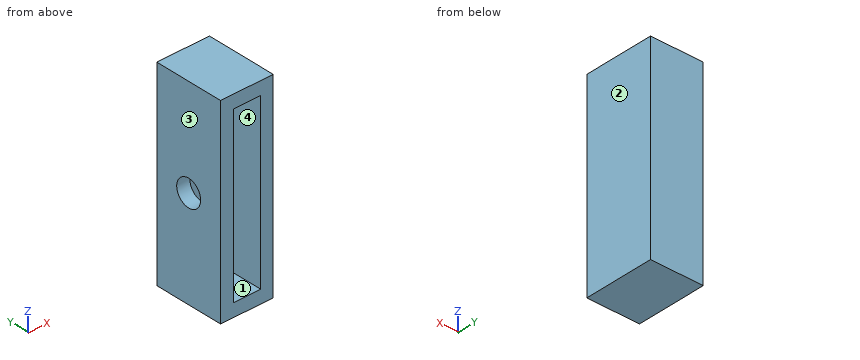
from build123d import *

# Parameters (mm, degrees)
F0_W     = 304.8
F0_H     = 1143
F1_DEPTH = 406.4
F2_W     = 156.097188
F2_H     = 990.6
F3_DEPTH = 381
F4_R     = 76.2
F5_DEPTH = 76.2


with BuildPart() as f1:
    # F0 (on Front) → F1 (new body)
    with BuildSketch(Plane.XZ):
        Rectangle(F0_W, F0_H)
    extrude(amount=F1_DEPTH)

    # F2 (on face) → F3 (cut)
    with BuildSketch(Plane.XZ.offset(406.4)):
        with Locations((1.848594, 0)):
            Rectangle(F2_W, F2_H)
    extrude(amount=-F3_DEPTH, mode=Mode.SUBTRACT)

    # F4 (on face) → F5 (cut)
    with BuildSketch(Plane(origin=(-152.4, 0, 0), x_dir=(0, -1, 0), z_dir=(-1, 0, 0))):
        with Locations((203.2, 0)):
            Circle(F4_R)
    extrude(amount=-F5_DEPTH, mode=Mode.SUBTRACT)


solid = f1.part
CAD build for the part. Positions are in the model's coordinates, mm. Face numbers are marked on the shaded views. Round coordinates to 2 decimals unless told otherwise and drop trailing zeros. Order: outer loops, then holes, each group sorted by start corner. A loop starts at its lowest first (then second) coordinate and runs counter-clockwise, first axis right, second up. Notation, with made-up numbers: (7.25, 15) -> (15.25, 15) arc R37 ccw to (15.25, 51) -> close; hole circle Ø3 at (40, -12). An arc over 180 degrees is marked (long way). Write item = value, one per line. Start each with the question number.
(1) Pull direction X, two halves, no side cores. Call the marked faces 1, 2, 3 and 4: released by +X, released by -X, zero draft, split by the parting line, or undercut.
(2) Probe line 1 (X direction, y = -309, z = -451); line 2 (Z direction, x = -56, y = -90); line 3 (Z direction, x = -123, y = -203.2). List the from-to ranges inside material, lowest first. Write a range as [from, to].
(3) Cut at A-A, the plane z = 0. List the corners of the cut face in (x, y), then the cut area to 3 significant figures.
(4) Cut at C-C, the plane x = 5.5. List the corners of the cut face in (y, z), then the cut area to 3 significant figures.
(5) Cut at D-D, the plane y = -203.2. List the corners of the cut face in (x, z).
(6) Cut at B-B, the plane y = -105. List the corners of the cut face in (x, z), then the cut area to 3 significant figures.
Model answer:
q1.face_1 = undercut
q1.face_2 = released by +X
q1.face_3 = released by -X
q1.face_4 = undercut
q2.line_1 = [-152.4, -76.2], [79.9, 152.4]
q2.line_2 = [-571.5, -495.3], [495.3, 571.5]
q2.line_3 = [-571.5, -76.2], [76.2, 571.5]
q3.outline = (-152.4, -406.4) -> (-76.2, -406.4) -> (-76.2, -279.4) -> (-152.4, -279.4) -> close; (-152.4, -127) -> (-76.2, -127) -> (-76.2, -25.4) -> (79.9, -25.4) -> (79.9, -406.4) -> (152.4, -406.4) -> (152.4, 0) -> (-152.4, 0) -> close
q3.area = 52,800 mm2
q4.outline = (-406.4, -571.5) -> (0, -571.5) -> (0, 571.5) -> (-406.4, 571.5) -> (-406.4, 495.3) -> (-25.4, 495.3) -> (-25.4, -495.3) -> (-406.4, -495.3) -> close
q4.area = 87,100 mm2
q5.outline = (-152.4, -571.5) -> (152.4, -571.5) -> (152.4, 571.5) -> (-152.4, 571.5) -> (-152.4, 76.2) -> (-76.2, 76.2) -> (-76.2, 495.3) -> (79.9, 495.3) -> (79.9, -495.3) -> (-76.2, -495.3) -> (-76.2, -76.2) -> (-152.4, -76.2) -> close
q6.outline = (-152.4, -571.5) -> (152.4, -571.5) -> (152.4, 571.5) -> (-152.4, 571.5) -> close; hole (-76.2, -495.3) -> (79.9, -495.3) -> (79.9, 495.3) -> (-76.2, 495.3) -> close
q6.area = 194,000 mm2
